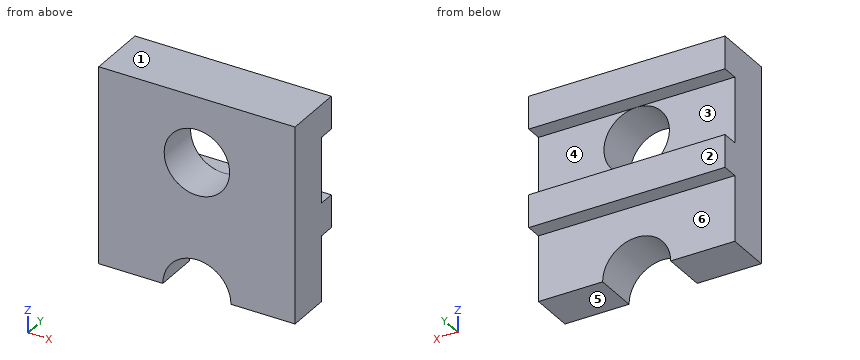
from build123d import *

# Parameters (mm, degrees)
SKETCH1_W           = 9.525
SKETCH1_H           = 9.525
BOSS_EXTRUDE1_DEPTH = 2.921
SKETCH2_W           = 9.525
SKETCH2_H           = 3.175
CUT_EXTRUDE1_DEPTH  = 0.7874
SKETCH3_R           = 1.5875
CUT_EXTRUDE2_DEPTH  = 8.065059197


with BuildPart() as part:
    # Sketch1 → Boss-Extrude1 (new body)
    with BuildSketch(Plane(origin=(0, 0, 0), x_dir=(1, 0, 0), z_dir=(0, 1, 0))):
        Rectangle(SKETCH1_W, SKETCH1_H)
    extrude(amount=BOSS_EXTRUDE1_DEPTH)

    # Sketch2 → Cut-Extrude1 (cut)
    with BuildSketch(Plane(origin=(0, 2.921, 0), x_dir=(1, 0, 0), z_dir=(0, 1, 0))):
        with Locations((0, -1.5875)):
            Rectangle(SKETCH2_W, SKETCH2_H)
        with Locations((0, 3.175)):
            Rectangle(SKETCH2_W, SKETCH2_H)
    extrude(amount=-CUT_EXTRUDE1_DEPTH, mode=Mode.SUBTRACT)

    # Sketch3 → Cut-Extrude2 (cut, through all)
    with BuildSketch(Plane(origin=(0, 2.1336, 0), x_dir=(1, 0, 0), z_dir=(0, 1, 0))):
        with Locations(Location((0, -1.5875, 0), (0, 0, 270))):
            Circle(SKETCH3_R)
        with BuildLine():
            Line((-1.651, 4.7625), (1.651, 4.7625))
            ThreePointArc((1.651, 4.7625), (0, 3.1115), (-1.651, 4.7625))
        make_face()
    extrude(amount=-CUT_EXTRUDE2_DEPTH, mode=Mode.SUBTRACT)


solid = part.part
Build history of the part. All positions in model axes, mm. Face numbers are marked on the shaded views. A direction names the side the tool comes from. Round coordinates to 2 decimals unless told otherwise and drop trailing zeros. Write each loop counter-clockwise with the first axis right and the second up, starting at its lowest first coordinate (ties: lowest second). Pieces come first, ordered by that corner, then holes. Notation, with made-up numbers: (50.5, 19) -> (54.5, 19) arc R14 ccw to (54.5, 26) -> close; hole circle Ø3 at (-12.75, 21.5). An arc over 180 degrees is marked (long way). Use one line per item in the form item = value.
Q1. Drill centre lines: L1, parallel to Z at x = 0, y = 1.4 (1 decimal); L2, parallel to X at y = 0.6, z = 1.5; L3, parallel to Z at x = -3, y = 2.45 (1 decimal). Where is each one in solid material? Low to high.
Conclusion:
L1 = -3.1 to 0, 3.2 to 4.8
L2 = -4.76 to -1.59, 1.59 to 4.76
L3 = -1.6 to 0, 3.2 to 4.8
Q2. Band-saw the part on B-B, the plane z = 0.5. Write the cut outline in (x, y), then the cut area to 3 significant figures.
Conclusion:
outline = (-4.76, 0) -> (-1.16, 0) -> (-1.16, 2.13) -> (-4.76, 2.13) -> close; (1.16, 0) -> (4.76, 0) -> (4.76, 2.13) -> (1.16, 2.13) -> close
area = 15.4 mm²
Q3. Drop flat-ended pins along their axis: P1, Ø0.6, axis at x = 1.5, y = 2.5, coming from the -Z side; P2, Ø2.5, axis at x = -0.5, z = -3.5, coming from the +Y side. Give the stop position or say it passes through.
Conclusion:
P1 = -1.59
P2 = 2.13
Q4. Band-saw the part on D-D, the plane z = 3. Write the cut outline in (x, y), then the cut area to 3 significant figures.
Conclusion:
outline = (-4.76, 0) -> (-0.72, 0) -> (-0.72, 2.13) -> (-4.76, 2.13) -> close; (0.72, 0) -> (4.76, 0) -> (4.76, 2.13) -> (0.72, 2.13) -> close
area = 17.2 mm²
Q5. Tool access for the marked faces 5 and 6: list every direction of +Z, -Z, +X, -X, +Y, -Y with a clear straight run to the whole face (end or side of a thin tool).
Conclusion:
face_5 = -Z, +X, -X, +Y, -Y
face_6 = -Z, +X, -X, +Y
Q6. Band-saw the part on A-A, the plane y = 1.1. Write the cut outline in (x, z) (1 decimal), then the cut area to 3 significant figures.
Conclusion:
outline = (-4.8, -4.8) -> (-1.7, -4.8) arc R1.7 cw to (1.7, -4.8) -> (4.8, -4.8) -> (4.8, 4.8) -> (-4.8, 4.8) -> close; hole circle Ø3.2 at (0, 1.6)
area = 78.5 mm²
Q7. Two-plate mould, pull along Z, no slides. Class the marked faces 1, 2, 3 and 4: released by +Z, released by -Z, zero draft, split by the parting line, or undercut.
Conclusion:
face_1 = released by +Z
face_2 = zero draft
face_3 = undercut
face_4 = undercut
